CAD build for the part. Positions are in the model's coordinates, mm. A direction names the side the tool comes from. Round coordinates to 2 decimals unless told otherwise and drop trailing zeros. Loops run counter-clockwise (first coordinate to the right, second up) from the corner with the lowest first, then second, coordinate; pieces in that order, holes last. Notation, with made-up numbers: (-33.75, -4) - (-15.75, -4) arc R15 cw to (-15.75, 4) - close; hole circle Ø1 at (-22.75, 75.5). An arc over 180 degrees is marked (long way). One line per question, with ' | ' between items.
```python
from build123d import *

# Parameters (mm, degrees)
F0_R     = 13
F1_DEPTH = 30
F2_R     = 11.5
F3_DEPTH = 25
F4_W     = 4
F4_H     = 8
F5_DEPTH = 20
F7_DEPTH = 4


with BuildPart() as f1:
    # F0 (on Front) → F1 (new body)
    with BuildSketch(Plane.XZ):
        Circle(F0_R)
    extrude(amount=F1_DEPTH)

    # F2 (on Front) → F3 (cut)
    with BuildSketch(Plane.XZ):
        Circle(F2_R)
    extrude(amount=F3_DEPTH, mode=Mode.SUBTRACT)

    # F4 (on face) → F5 (join)
    with BuildSketch(Plane.XZ.offset(30)):
        with Locations((0, 16.845233)):
            Rectangle(F4_W, F4_H)
    extrude(amount=-F5_DEPTH)

    # F6 (on face) → F7 (cut)
    with BuildSketch(Plane.YZ.offset(2)):
        Polygon((-10, 20.845233), (-20, 20.845233), (-10, 14.845233), align=None)
    extrude(amount=-F7_DEPTH, mode=Mode.SUBTRACT)


solid = f1.part
```
(1) Probe L1, parallel to Z at x = 0, y = -6.25; L2, parallel to X at y = -7.75, z = 7; L3, parallel to Z at x = 3.5, y = -4. List the from-to ranges inside material, lowest first.
Results found:
L1: z = -13 to -11.5, 11.5 to 13 | L2: x = -10.95 to -9.12, 9.12 to 10.95 | L3: z = -12.52 to -10.95, 10.95 to 12.52
(2) Drop flat-ended pins along their axis: P1, Ø1.5, axis at x = -9, z = 2, coming from the +Y side; P2, Ø12, axis at y = -17, z = -6.5, coming from the -X side; P3, Ø3, axis at x = 4, y = -6.5, coming from the -Z side. Give the stop position or say it passes through.
Results found:
P1: stops at y = -25 | P2: stops at x = -12.99 | P3: stops at z = -12.76
(3) Two-plate mould, pull along Z, no slides. Class faces 4 (the face through (0, -25, 20.845)), 5 (the face through (-1.5, -12.3, 11.4)), 6 (the face through (0, -25, 0)), 7 (the face through (0, -10, 14)): released by +Z, released by -Z, zero draft, split by the parting line, or undercut.
Results found:
face 4: released by +Z | face 5: undercut | face 6: undercut | face 7: zero draft
(4) Cut at D-D, the plane x = -7.5. Write the cut outline in (y, z), then the cut area to 3 significant figures.
Results found:
outline: (-30, -10.62) - (0, -10.62) - (0, -8.72) - (-25, -8.72) - (-25, 8.72) - (0, 8.72) - (0, 10.62) - (-30, 10.62) - close | area: 201 mm²
(5) Cut at A-A, the plane x = 0. Write the cut outline in (y, z), then the cut area to 3 significant figures.
Results found:
outline: (-30, -13) - (0, -13) - (0, -11.5) - (-25, -11.5) - (-25, 11.5) - (0, 11.5) - (0, 13) - (-10, 13) - (-10, 14.85) - (-20, 20.85) - (-30, 20.85) - close | area: 332 mm²
(6) Cut at B-B, the plane y = -22. Write the cut outline in (x, z).
Results found:
outline: (-2, 12.85) arc R13 ccw (long way) to (2, 12.85) - (2, 20.85) - (-2, 20.85) - close; hole circle Ø23 at (0, 0)
(7) Tool access for faces 1 (the face through (2, -22, 17)), 2 (the face through (0.028, -15.07, 17.887)), 3 (the face through (-2, -22, 17)): list every direction of +Z, -Z, +X, -X, +Y, -Y with a clear straight run to the whole face (end or side of a thin tool).
Results found:
face 1: +Z, +X, +Y, -Y | face 2: +Z, +X, -X, +Y | face 3: +Z, -X, +Y, -Y
(8) Cut at C-C, the plane z = 0. Write the cut outline in (x, y).
Results found:
outline: (-13, -30) - (13, -30) - (13, 0) - (11.5, 0) - (11.5, -25) - (-11.5, -25) - (-11.5, 0) - (-13, 0) - close
